Geometry: see drawing. Coordinates: mm, zero at the bounding-box minimum. A direction names the side the tool comes from. Round coordinates to 2 decimals unless told otherwise and drop trailing zeros. Order: outer loops, then holes, each group sorted by start corner. A loop starts at its lowest first (then second) coordinate and runs counter-clockwise, first axis right, second up. Notation, with made-up numbers: (15, -11) -> (67, -11) arc R24 cw to (67, 21) -> close; hole circle Ø11 at (-2.75, -15). An arc over 180 degrees is marked (long way). One line per item, written item: value. Start each with the question number.
1) Reachability of the marked faces 1, 2 and 3 from +Z, -Z, +X, -X, +Y, -Y: full face, straight path, thin tool, end or side. Return the list, or none.
2) Section C-C (x = 5.5). Return the cut outline in (y, z) (1 decimal), and give its area (3 significant figures).
3) Pin query (flat end, axial travel): P1, Ø8, axis at x = 9.5, z = 6.5, coming from the -Y side; P2, Ø1, axis at x = 12.5, z = 16, coming from the +Y side (1 decimal); P3, Ø4, axis at x = 7.33, y = 6.35, coming from the +Z side; P4, Ø1.5, axis at y = 5, z = 5.5, coming from the +X side. Return the tip coordinate at first contact, or that it passes through.
4) Mould query, pull axis Y, two halves, no side actions, for the marked faces 4, 5 and 6. Classes: pulls with the +Y half, pulls with the -Y half, needs draft (parallel to the pull), parting line crosses it, or undercut.
5) Ray query, L1, parallel to Z at x = 9, y = 10 (1 decimal); L2, parallel to X at y = 5.5, z = 22.25 (1 decimal); L3, parallel to X at y = 4.75, z = 15 (1 decimal). Return the intervals inside material, ascending.
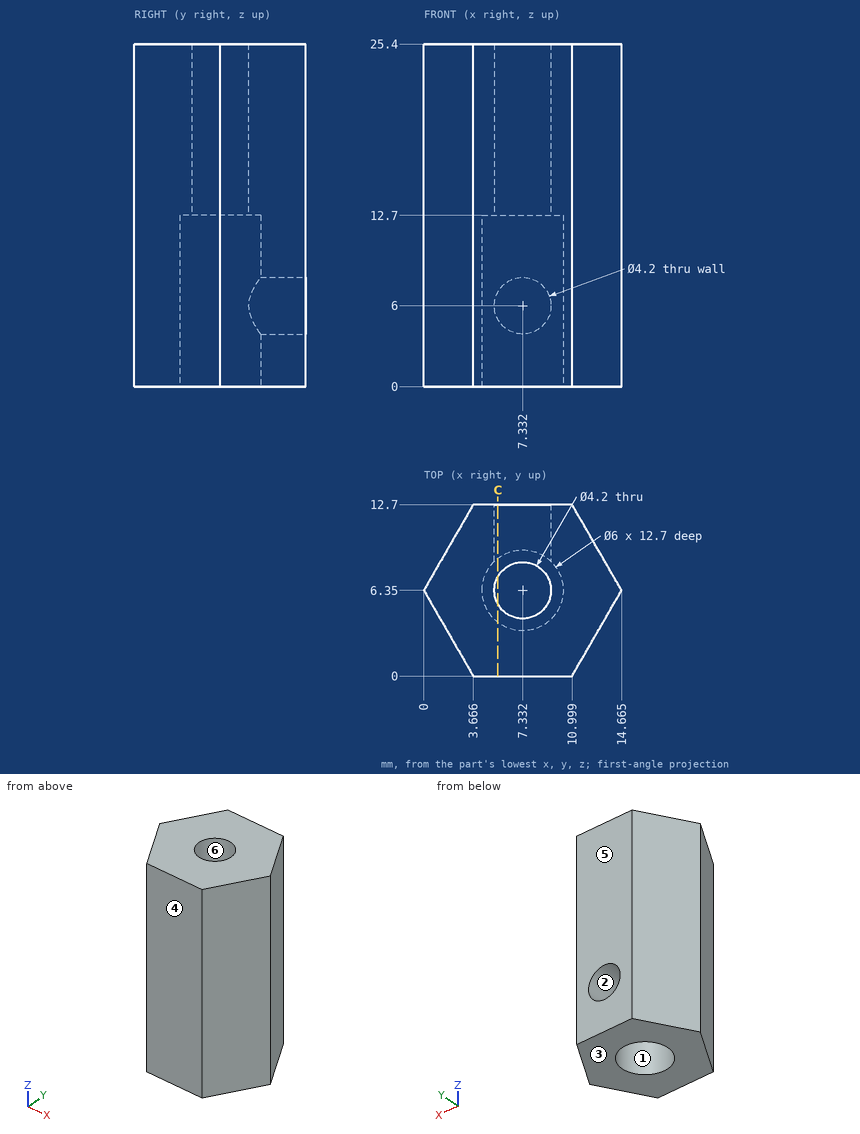
Findings:
1. face 1: -Z
1. face 2: +Y
1. face 3: -Z, +X, -X, +Y, -Y
2. outline: (0, 0) -> (4, 0) -> (4, 12.7) -> (5.3, 12.7) -> (5.3, 25.4) -> (0, 25.4) -> close; (7.4, 12.7) -> (8.7, 12.7) -> (8.7, 7) -> (12.7, 7) -> (12.7, 25.4) -> (7.4, 25.4) -> close; (8.7, 0) -> (12.7, 0) -> (12.7, 5) -> (8.7, 5) -> close
2. area: 228 mm2
3. P1: y = 0
3. P2: y = 11
3. P3: through
3. P4: x = 14.32
4. face 4: pulls with the -Y half
4. face 5: pulls with the +Y half
4. face 6: undercut
5. L1: 0 to 4.7, 7.3 to 25.4
5. L2: 0.5 to 5.4, 9.3 to 14.2
5. L3: 0.9 to 6, 8.7 to 13.7
